```python
from build123d import *

# Parameters (mm, degrees)
SKETCH_1_W         = 10
SKETCH_1_H         = 5.1
EXTRUDE_1_DEPTH    = 2
EXTRUDE_1_2_DEPTH  = 2
SKETCH_2_W         = 66
SKETCH_2_H         = 20
EXTRUDE_2_DEPTH    = 3
HOLE_WIZARD_M4_1_D = 4.8
CHAMFER_1_SIZE     = 1


with BuildPart() as part:
    # Sketch 1 → Extrude 1 (new body)
    with BuildSketch(Plane.XY):
        with Locations((28, 0)):
            Rectangle(SKETCH_1_W, SKETCH_1_H)
    extrude(amount=EXTRUDE_1_DEPTH)



with BuildPart() as body_2:
    # Sketch 1 → Extrude 1 2 (new body)
    with BuildSketch(Plane.XY):
        with Locations((-28, 0)):
            Rectangle(SKETCH_1_W, SKETCH_1_H)
    extrude(amount=EXTRUDE_1_2_DEPTH)


with BuildPart() as part_1:
    add(part.part)

    add(body_2.part)  # Extrude 2 merges body 2
    # Sketch 2 → Extrude 2 (add)
    with BuildSketch(Plane.XY.offset(2)):
        Rectangle(SKETCH_2_W, SKETCH_2_H)
    extrude(amount=EXTRUDE_2_DEPTH)

    # Hole Wizard M4 _ _1 (through all)
    with Locations(Plane.XY.offset(5)):
        with Locations((-28, 0), (28, 0)):
            Hole(HOLE_WIZARD_M4_1_D / 2)

    # Chamfer 1
    chamfer_1_edges = [part_1.edges().sort_by_distance(p)[0] for p in [
        (-33, 0, 5),
        (0, -10, 5),
        (33, 0, 5),
        (0, 10, 5),
    ]]
    chamfer(chamfer_1_edges, length=CHAMFER_1_SIZE)


solid = part_1.part
```
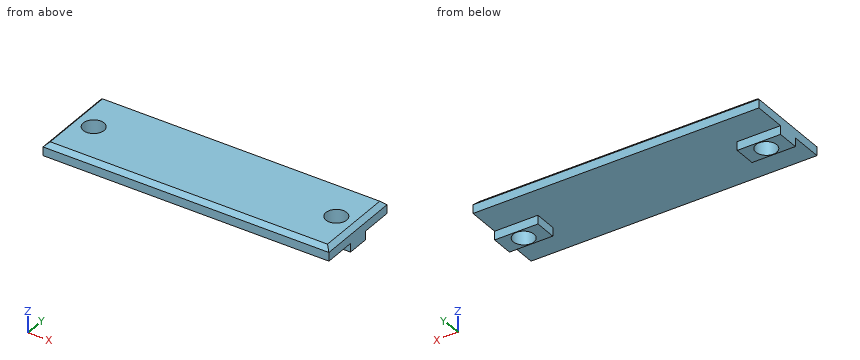
Geometry check sheet. Reference: the model listing, model coordinates, mm. Round coordinates to 2 decimals unless told otherwise and drop trailing zeros. Loops run counter-clockwise (first coordinate to the right, second up) from the corner with the lowest first, then second, coordinate; pieces in that order, holes last. Notation, with made-up numbers: (15.25, 87.5) - (27.25, 87.5) arc R32 cw to (27.25, 117.5) - close; hole circle Ø1 at (24.25, 37.5). An arc over 180 degrees is marked (long way). Write item = value, one per line. Start each with the question number.
1. Section check B-B on y = 0. Enter the section's corners in (x, z).
2. Section check A-A on z = 0.9. Enter the section's corners in (x, y), then the cut area to 3 significant figures.
3. Section check D-D on x = -19. Enter the section's corners in (y, z).
4. Thickness scan on line 1 (X direction, y = 0.25, z = 2.25); line 2 (Y direction, x = 28, z = 1.5); line 3 (X direction, y = -0.5, z = 0.95). Record the ranges inside material, lowest first.
5. Section check C-C on x = -28. Enter the section's corners in (y, z).
6. Depth check by flat-ended pin: pin 1 (4.5 mm diameter, centred on x = 28, y = 0, fed in from +Z); pin 2 (1 mm diameter, centred on x = 2, y = -5, fed in from -Z); pin 3 (0.6 mm diameter, centred on x = 28.5, z = 0.5, fed in from +Y); pin 4 (0.6 mm diameter, centred on x = 29, z = 1.5, fed in from -Y). Enter the tip coordinate at first touch or a pass-through.
Working result:
q1.outline = (-33, 0) - (-30.4, 0) - (-30.4, 5) - (-32, 5) - (-33, 4) - close; (-25.6, 0) - (-23, 0) - (-23, 2) - (23, 2) - (23, 0) - (25.6, 0) - (25.6, 5) - (-25.6, 5) - close; (30.4, 0) - (33, 0) - (33, 4) - (32, 5) - (30.4, 5) - close
q2.outline = (-33, -2.55) - (-23, -2.55) - (-23, 2.55) - (-33, 2.55) - close; (23, -2.55) - (33, -2.55) - (33, 2.55) - (23, 2.55) - close; hole circle Ø4.8 at (-28, 0); hole circle Ø4.8 at (28, 0)
q2.area = 65.8 mm^2
q3.outline = (-10, 2) - (10, 2) - (10, 4) - (9, 5) - (-9, 5) - (-10, 4) - close
q4.line_1 = -33 to -30.39, -25.61 to 25.61, 30.39 to 33
q4.line_2 = -2.55 to -2.4, 2.4 to 2.55
q4.line_3 = -33 to -30.35, -25.65 to -23, 23 to 25.65, 30.35 to 33
q5.outline = (-10, 2) - (-2.55, 2) - (-2.55, 0) - (-2.4, 0) - (-2.4, 5) - (-9, 5) - (-10, 4) - close; (2.4, 0) - (2.55, 0) - (2.55, 2) - (10, 2) - (10, 4) - (9, 5) - (2.4, 5) - close
q6.pin_1 = through
q6.pin_2 = 2
q6.pin_3 = 2.55
q6.pin_4 = -2.55
